Work out the finished part from the listing and answer in its coordinate system (mm). A direction names the side the tool comes from. Round coordinates to 2 decimals unless told otherwise and drop trailing zeros. Loops run counter-clockwise (first coordinate to the right, second up) from the corner with the lowest first, then second, coordinate; pieces in that order, holes last. Notation, with made-up numbers: (-16, 15) -> (10, 15) arc R22 cw to (10, 30) -> close; hole circle Ø10 at (13, 1.5). An arc over 180 degrees is marked (long way). Use CSV: the item, a comma, the result in double quotes. Start each with the question number.
from build123d import *

# Parameters (mm, degrees)
SKETCH1_R           = 2.5
BOSS_EXTRUDE2_DEPTH = 4
BOSS_EXTRUDE3_DEPTH = 11
SKETCH4_R           = 11
CUT_EXTRUDE1_DEPTH  = 6
SKETCH5_R           = 10
BOSS_EXTRUDE5_DEPTH = 10
SKETCH6_W           = 5.8
SKETCH6_H           = 2.8
CUT_EXTRUDE2_DEPTH  = 8.8
SKETCH8_R           = 1.6
CUT_EXTRUDE3_DEPTH  = 10
SKETCH10_R          = 3.1
CUT_EXTRUDE5_DEPTH  = 103.102889283
SKETCH11_R          = 2.25
CUT_EXTRUDE6_DEPTH  = 10
CUT_EXTRUDE7_DEPTH  = 2


with BuildPart() as part:
    # Sketch1 → Boss-Extrude2 (new body)
    with BuildSketch(Plane(origin=(0, 0, 0), x_dir=(1, 0, 0), z_dir=(0, 1, 0))):
        with BuildLine():
            Line((-10, 0), (-60, 0))
            ThreePointArc((-60, 0), (-67.071067812, 2.928932188), (-70, 10))
            Line((-70, 10), (-70, 60))
            ThreePointArc((-70, 60), (-67.071067812, 67.071067812), (-60, 70))
            Line((-60, 70), (-10, 70))
            ThreePointArc((-10, 70), (-2.928932188, 67.071067812), (0, 60))
            Line((0, 60), (0, 10))
            ThreePointArc((0, 10), (-2.928932188, 2.928932188), (-10, 0))
        make_face()
        with Locations(Location((-50.25, 50.25, 0), (0, 0, 270))):
            Circle(SKETCH1_R, mode=Mode.SUBTRACT)
        with Locations(Location((-29.56712665, 29.56712665, 0), (0, 0, 270))):
            Circle(SKETCH1_R, mode=Mode.SUBTRACT)
    extrude(amount=BOSS_EXTRUDE2_DEPTH)

    # Sketch2 → Boss-Extrude3 (add)
    with BuildSketch(Plane(origin=(0, 4, 0), x_dir=(1, 0, 0), z_dir=(0, 1, 0))):
        with BuildLine():
            Line((-10, 0), (-60, 0))
            ThreePointArc((-60, 0), (-67.071067812, 2.928932188), (-70, 10))
            Line((-70, 10), (-70, 60))
            ThreePointArc((-70, 60), (-67.071067812, 67.071067812), (-60, 70))
            Line((-60, 70), (-10, 70))
            ThreePointArc((-10, 70), (-2.928932188, 67.071067812), (0, 60))
            Line((0, 60), (0, 10))
            ThreePointArc((0, 10), (-2.928932188, 2.928932188), (-10, 0))
        make_face()
        with BuildLine():
            Line((-3, 13), (-3, 57))
            ThreePointArc((-3, 57), (-5.928932188, 64.071067812), (-13, 67))
            Line((-13, 67), (-57, 67))
            ThreePointArc((-57, 67), (-64.071067812, 64.071067812), (-67, 57))
            Line((-67, 57), (-67, 13))
            ThreePointArc((-67, 13), (-64.071067812, 5.928932188), (-57, 3))
            Line((-57, 3), (-13, 3))
            ThreePointArc((-13, 3), (-5.928932188, 5.928932188), (-3, 13))
        make_face(mode=Mode.SUBTRACT)
    extrude(amount=BOSS_EXTRUDE3_DEPTH)

    # Sketch4 → Cut-Extrude1 (cut)
    with BuildSketch(Plane(origin=(0, 4, 0), x_dir=(1, 0, 0), z_dir=(0, 1, 0))):
        with Locations(Location((-50.25, 50.25, 0), (0, 0, 270))):
            Circle(SKETCH4_R)
    extrude(amount=-CUT_EXTRUDE1_DEPTH, mode=Mode.SUBTRACT)

    # Sketch5 → Boss-Extrude5 (add)
    with BuildSketch(Plane.XZ):
        with Locations(Location((-29.56712665, -29.56712665, 0), (0, 0, 90))):
            Circle(SKETCH5_R)
    extrude(amount=BOSS_EXTRUDE5_DEPTH)

    # Sketch6 → Cut-Extrude2 (cut)
    with BuildSketch(Plane.XZ.offset(10)):
        with Locations((-29.56712665, -36.06712665)):
            Rectangle(SKETCH6_W, SKETCH6_H)
    extrude(amount=-CUT_EXTRUDE2_DEPTH, mode=Mode.SUBTRACT)

    # Sketch8 → Cut-Extrude3 (cut)
    with BuildSketch(Plane(origin=(-29.56712665, -10, -39.56712665), x_dir=(-1, 0, 0), z_dir=(0, 0, -1))):
        with Locations((0, 5)):
            Circle(SKETCH8_R)
    extrude(amount=-CUT_EXTRUDE3_DEPTH, mode=Mode.SUBTRACT)

    # Sketch10 → Cut-Extrude5 (cut, through all)
    with BuildSketch(Plane.XZ.offset(10)):
        with Locations(Location((-29.56712665, -29.56712665, 0), (0, 0, 270))):
            Circle(SKETCH10_R)
    extrude(amount=-CUT_EXTRUDE5_DEPTH, mode=Mode.SUBTRACT)

    # Sketch11 → Cut-Extrude6 (cut)
    with BuildSketch(Plane(origin=(0, 4, 0), x_dir=(1, 0, 0), z_dir=(0, 1, 0))):
        with Locations(Location((-8, 62, 0), (0, 0, 270))):
            Circle(SKETCH11_R)
        with Locations(Location((-62, 62, 0), (0, 0, 270))):
            Circle(SKETCH11_R)
        with Locations(Location((-62, 8, 0), (0, 0, 270))):
            Circle(SKETCH11_R)
        with Locations(Location((-8, 8, 0), (0, 0, 270))):
            Circle(SKETCH11_R)
    extrude(amount=-CUT_EXTRUDE6_DEPTH, mode=Mode.SUBTRACT)

    # Sketch12 → Cut-Extrude7 (cut)
    with BuildSketch(Plane.XZ):
        Polygon((-62, -3.669872981), (-65.75, -5.834936491), (-65.75, -10.165063509), (-62, -12.330127019), (-58.25, -10.165063509), (-58.25, -5.834936491), align=None)
        Polygon((-8, -3.669872981), (-11.75, -5.834936491), (-11.75, -10.165063509), (-8, -12.330127019), (-4.25, -10.165063509), (-4.25, -5.834936491), align=None)
        Polygon((-62, -57.669872981), (-65.75, -59.834936491), (-65.75, -64.165063509), (-62, -66.330127019), (-58.25, -64.165063509), (-58.25, -59.834936491), align=None)
        Polygon((-8, -57.669872981), (-11.75, -59.834936491), (-11.75, -64.165063509), (-8, -66.330127019), (-4.25, -64.165063509), (-4.25, -59.834936491), align=None)
    extrude(amount=-CUT_EXTRUDE7_DEPTH, mode=Mode.SUBTRACT)


solid = part.part
Q1. Section A-A, the plane y = 13.75 is taken. Write down the section's boundary in (x, z), and give its area (3 significant figures).
Q2. Section C-C, the plane z = -29 is taken. Write down the section's boundary in (x, y), and give its area (3 significant figures).
Q3. For a pull along Z with two mould halves and no side action, classify faces 4 (the flat face through (-9.85, 0.99, -58.74)), 5 (the flat face through (-35, 7, 0)), 6 (the cylindrical face through (-31.093, -4.519, -33.462)) as pulls with the +Z half, pulls with the -Z half, needs draft (parallel to the pull), parting line crosses it, or undercut.
Q4. Section B-B, the plane x = -56 is taken. Write down the section's boundary in (y, z), and give its area (3 significant figures).
Q5. Which of the six approach directions +Z, -Z, +X, -X, +Y, -Y give full straight-line access (tool end or side, diameter ignored) to faces 1 (the flat face through (0, 7, -35)), 2 (the flat face through (-32.467, -6, -36)), 3 (the flat face through (-67, 9, -35))?
Q6. Each of these flat-tipped pins is pushed along its axis until it touches: pin 1 (2 mm diameter, centred on x = -63, z = -63.5, fed in from -Y); pin 2 (4 mm diameter, centred on x = -62, z = -62, fed in from +Y); pin 3 (0.6 mm diameter, centred on y = 0.5, z = -61.5, fed in from -X); pin 4 (1 mm diameter, centred on y = 0.5, z = -8.5, fed in from +X). Where does it stop, or does it pass through?
Q7. Section D-D, the plane z = -8 is taken. Write down the section's boundary in (x, y).
Q8. Straight lines are drawn through the part: line 1 (Z direction, x = -42, y = 12.5); line 2 (Z direction, x = -62.5, y = 1). For each, find the intervals that lie inside material, in ascending order. Write a range as from..to.
Report:
1,outline,"(-70, -60) arc R10 ccw to (-60, -70) -> (-10, -70) arc R10 ccw to (0, -60) -> (0, -10) arc R10 ccw to (-10, 0) -> (-60, 0) arc R10 ccw to (-70, -10) -> close; hole (-67, -57) arc R10 ccw to (-57, -67) -> (-13, -67) arc R10 ccw to (-3, -57) -> (-3, -13) arc R10 ccw to (-13, -3) -> (-57, -3) arc R10 ccw to (-67, -13) -> close"
1,area,"804 mm²"
2,outline,"(-70, 0) -> (-39.55, 0) -> (-39.55, -10) -> (-32.61, -10) -> (-32.61, 4) -> (-67, 4) -> (-67, 15) -> (-70, 15) -> close; (-26.52, -10) -> (-19.58, -10) -> (-19.58, 0) -> (0, 0) -> (0, 15) -> (-3, 15) -> (-3, 4) -> (-26.52, 4) -> close"
2,area,"460 mm²"
3,face 4,"undercut"
3,face 5,"pulls with the +Z half"
3,face 6,"needs draft"
4,outline,"(0, -70) -> (15, -70) -> (15, -67) -> (4, -67) -> (4, -59.63) -> (0, -59.63) -> close; (0, -40.87) -> (4, -40.87) -> (4, -3) -> (15, -3) -> (15, 0) -> (0, 0) -> close"
4,area,"271 mm²"
5,face 1,"+Z, -Z, +X, +Y, -Y"
5,face 2,"-Y"
5,face 3,"+Y"
6,pin 1,"stops at y = 2"
6,pin 2,"passes through"
6,pin 3,"stops at x = -69.93"
6,pin 4,"stops at x = -0.05"
7,outline,"(-69.8, 0) -> (-65.75, 0) -> (-65.75, 2) -> (-64.25, 2) -> (-64.25, 4) -> (-65.66, 4) -> (-65.66, 15) -> (-69.8, 15) -> close; (-59.75, 2) -> (-58.25, 2) -> (-58.25, 0) -> (-11.75, 0) -> (-11.75, 2) -> (-10.25, 2) -> (-10.25, 4) -> (-59.75, 4) -> close; (-5.75, 2) -> (-4.25, 2) -> (-4.25, 0) -> (-0.2, 0) -> (-0.2, 15) -> (-4.34, 15) -> (-4.34, 4) -> (-5.75, 4) -> close"
8,line 1,"z = -70..-67, -3..0"
8,line 2,"z = -69.68..-66.04, -57.96..-12.04, -3.96..-0.32"
